from build123d import *

# Parameters (mm, degrees)
SKETCH_1_R          = 2.5
EXTRUDE_1_DEPTH     = 45
EXTRUDE_2_DEPTH     = 8
EXTRUDE_3_DEPTH     = 8
CHAMFER_1_SIZE      = 1
SKETCH_4_R          = 1.25
CUT_EXTRUDE_1_DEPTH = 8
CUT_EXTRUDE_START   = 8
SKETCH_5_R          = 1.25
CUT_EXTRUDE_2_DEPTH = 8


with BuildPart() as part:
    # 草图1 → 凸台-拉伸1 (new body)
    with BuildSketch(Plane(origin=(0, 0, 0), x_dir=(1, 0, 0), z_dir=(0, 1, 0))):
        with Locations(Location((0, 0, 0), (0, 0, 90))):
            Circle(SKETCH_1_R)
    extrude(amount=EXTRUDE_1_DEPTH)

    # 草图2 → 凸台-拉伸2 (add)
    with BuildSketch(Plane(origin=(0, 45, 0), x_dir=(1, 0, 0), z_dir=(0, 1, 0))):
        Polygon((3.202903935, -1.319623577), (2.744279509, 2.113984385), (-0.458624426, 3.433607962), (-3.202903935, 1.319623577), (-2.744279509, -2.113984385), (0.458624426, -3.433607962), align=None)
    extrude(amount=-EXTRUDE_2_DEPTH)

    # 草图3 → 凸台-拉伸3 (add)
    with BuildSketch(Plane.XZ):
        Polygon((3.202903935, 1.319623577), (0.458624426, 3.433607962), (-2.744279509, 2.113984385), (-3.202903935, -1.319623577), (-0.458624426, -3.433607962), (2.744279509, -2.113984385), align=None)
    extrude(amount=-EXTRUDE_3_DEPTH)

    # 倒角1
    # the kernel refuses this chamfer: 1 mm, written as the material it adds along each edge
    with BuildSketch(Plane(origin=(0, 37, 0), x_dir=(0, 0, -1), z_dir=(-1, 0, 0))) as chamfer_1_piece_1_section:
        Polygon((2.5, CHAMFER_1_SIZE), (2.5 + CHAMFER_1_SIZE, 0), (2.5, 0), align=None)
    chamfer_1_piece_1 = revolve(axis=Axis((0, 37, 0), (0, -1, 0)), mode=Mode.PRIVATE)
    chamfer_1_piece_1 = split(chamfer_1_piece_1, bisect_by=Plane(origin=(3.361202761, 36.482096178, 2.504767848), z_dir=(-0.9911972405355005, 0, 0.13239346794615373)), keep=Keep.TOP, mode=Mode.PRIVATE)
    chamfer_1_piece_1 = split(chamfer_1_piece_1, bisect_by=Plane(origin=(0.402796537, 36.482096178, 3.476613525), z_dir=(-0.61025472680424, 0, -0.7922052564917015)), keep=Keep.TOP, mode=Mode.PRIVATE)
    chamfer_1_piece_1 = split(chamfer_1_piece_1, bisect_by=Plane(origin=(2.183184145, 36.482096178, -2.345160432), z_dir=(-0.3809425137312606, 0, 0.924598724437855)), keep=Keep.TOP, mode=Mode.PRIVATE)
    chamfer_1_piece_1 = split(chamfer_1_piece_1, bisect_by=Plane(origin=(-0.102470937, 36.482096178, 3.202431915), z_dir=(0.38094251373126053, 0, -0.924598724437855)), keep=Keep.TOP, mode=Mode.PRIVATE)
    chamfer_1_piece_1 = split(chamfer_1_piece_1, bisect_by=Plane(origin=(-3.258731824, 36.482096178, -1.276618014), z_dir=(0.6102547268042401, 0, 0.7922052564917015)), keep=Keep.TOP, mode=Mode.PRIVATE)
    chamfer_1_piece_1 = split(chamfer_1_piece_1, bisect_by=Plane(origin=(-2.585980682, 36.482096178, 3.299128656), z_dir=(0.9911972405355005, 0, -0.1323934679461537)), keep=Keep.TOP, mode=Mode.PRIVATE)
    add(chamfer_1_piece_1)
    with BuildSketch(Plane(origin=(0, 8, 0), x_dir=(0, 0, -1), z_dir=(-1, 0, 0))) as chamfer_1_piece_2_section:
        Polygon((2.5 + CHAMFER_1_SIZE, 0), (2.5, -CHAMFER_1_SIZE), (2.5, 0), align=None)
    chamfer_1_piece_2 = revolve(axis=Axis((0, 8, 0), (0, -1, 0)), mode=Mode.PRIVATE)
    chamfer_1_piece_2 = split(chamfer_1_piece_2, bisect_by=Plane(origin=(0.402796537, 8.517903822, 3.476613525), z_dir=(-0.61025472680424, 0, -0.7922052564917015)), keep=Keep.TOP, mode=Mode.PRIVATE)
    chamfer_1_piece_2 = split(chamfer_1_piece_2, bisect_by=Plane(origin=(3.361202761, 8.517903822, 2.504767848), z_dir=(-0.9911972405355005, 0, 0.13239346794615373)), keep=Keep.TOP, mode=Mode.PRIVATE)
    chamfer_1_piece_2 = split(chamfer_1_piece_2, bisect_by=Plane(origin=(-0.102470937, 8.517903822, 3.202431915), z_dir=(0.38094251373126053, 0, -0.924598724437855)), keep=Keep.TOP, mode=Mode.PRIVATE)
    chamfer_1_piece_2 = split(chamfer_1_piece_2, bisect_by=Plane(origin=(2.183184145, 8.517903822, -2.345160432), z_dir=(-0.3809425137312606, 0, 0.924598724437855)), keep=Keep.TOP, mode=Mode.PRIVATE)
    chamfer_1_piece_2 = split(chamfer_1_piece_2, bisect_by=Plane(origin=(-2.585980682, 8.517903822, 3.299128656), z_dir=(0.9911972405355005, 0, -0.1323934679461537)), keep=Keep.TOP, mode=Mode.PRIVATE)
    chamfer_1_piece_2 = split(chamfer_1_piece_2, bisect_by=Plane(origin=(-3.258731824, 8.517903822, -1.276618014), z_dir=(0.6102547268042401, 0, 0.7922052564917015)), keep=Keep.TOP, mode=Mode.PRIVATE)
    add(chamfer_1_piece_2)

    # 草图4 → 切除-拉伸1 (cut)
    with BuildSketch(Plane(origin=(0, 0, 0), x_dir=(-1, 0, 0), z_dir=(0, 1, 0))):
        with Locations(Location((0, 0, 0), (0, 0, 90))):
            Circle(SKETCH_4_R)
    extrude(amount=CUT_EXTRUDE_1_DEPTH, mode=Mode.SUBTRACT)

    # 草图5 → 切除-拉伸2 (cut)
    with BuildSketch(Plane(origin=(0, 45, 0), x_dir=(-1, 0, 0), z_dir=(0, -1, 0)).offset(CUT_EXTRUDE_START)):
        with Locations(Location((0, 0, 0), (0, 0, 270))):
            Circle(SKETCH_5_R)
    extrude(amount=-CUT_EXTRUDE_2_DEPTH, mode=Mode.SUBTRACT)


solid = part.part
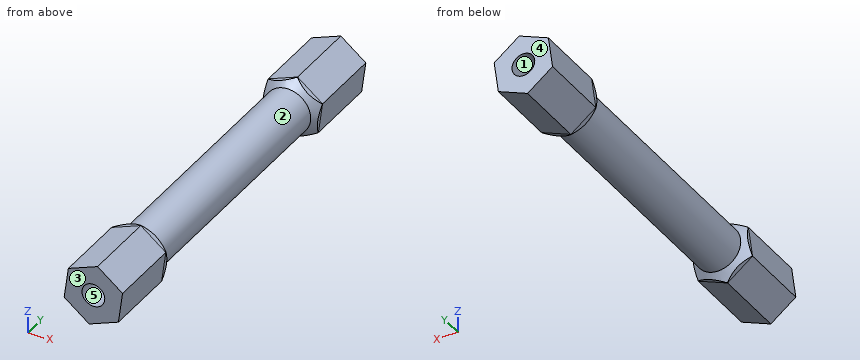
Design review of the part built by this model. Coordinates are the model's own, in mm. Face numbers are marked on the shaded views. A direction names the side the tool comes from. Give positions to 0.01 mm unless a question says otherwise; leave off trailing zeros. Write each loop counter-clockwise with the first axis right and the second up, starting at its lowest first coordinate (ties: lowest second). Pieces come first, ordered by that corner, then holes. Notation, with made-up numbers: M 74,42.5 L 131,42.5 A25 ccw 131,68.5 Z; hole C -7.75,14.5 d9. An arc over 180 degrees is marked long. Return JSON: item names as keys, results as strings. Group by question number.
Item 1: Take a section at B-B (x = 0). Give the boundary of the cut face in (y, z).
Item 2: Take a section at C-C (z = 0). Give the boundary of the cut face in (x, y), plus the area to 3 significant figures.
Item 3: The part is to be moulded in two halves that separate along X. For the marked faces 1, 2 and 3, say which applies: pulls with the +X half, pulls with the -X half, needs draft (parallel to the pull), parting line crosses it, or undercut.
Item 4: Clearance check with flat-ended pins moving along their axes: pin 1 Ø1.5 at (y, z) = (6, 1) entering from -X; pin 2 Ø2 at (x, z) = (0, 0) entering from +Y; pin 3 Ø3 at (x, y) = (0, 21.5) entering from +Z; pin 4 Ø3 at (x, z) = (0, 0) entering from -Y. State where each tip first meets the part, or that it passes through.
Item 5: Tool access review of the marked faces 4 and 5: name each direction out of +Z, -Z, +X, -X, +Y, -Y from which nothing blocks a thin tool from reaching the whole face with its end or side.
Item 6: Take a section at D-D (y = 19.5). Give the boundary of the cut face in (x, z), plus the area to 3 significant figures.
Item 7: Take a section at A-A (y = 7). Give the boundary of the cut face in (x, z), plus the area to 3 significant figures.
Item 8: Wall thickness on line 1 along X through (y, z) = (39.75, 0); line 2 along Y through (x, z) = (1, 0.5); line 3 along Y through (x, z) = (-2.5, 1.5): over which ranges is each line inside the solid? List them lowest first.
Return value:
{
 "1": {"outline": "M 0,-3.24 L 8.26,-3.24 L 9,-2.5 L 36,-2.5 L 36.74,-3.24 L 45,-3.24 L 45,-1.25 L 37,-1.25 L 37,1.25 L 45,1.25 L 45,3.24 L 36.74,3.24 L 36,2.5 L 9,2.5 L 8.26,3.24 L 0,3.24 L 0,1.25 L 8,1.25 L 8,-1.25 L 0,-1.25 Z"},
 "2": {"outline": "M -3.03,0 L -1.25,0 L -1.25,8 L 1.25,8 L 1.25,0 L 3.03,0 L 3.03,8.47 L 2.5,9 L 2.5,36 L 3.03,36.53 L 3.03,45 L 1.25,45 L 1.25,37 L -1.25,37 L -1.25,45 L -3.03,45 L -3.03,36.53 L -2.5,36 L -2.5,9 L -3.03,8.47 Z", "area": "203 mm2"},
 "3": {"face 1": "undercut", "face 2": "parting line crosses it", "face 3": "needs draft"},
 "4": {"pin 1": "stops at x = -2.99", "pin 2": "stops at y = 37", "pin 3": "stops at z = 2.5", "pin 4": "stops at y = 0"},
 "5": {"face 4": "+Z, -Z, +X, -X, +Y", "face 5": "-Y"},
 "6": {"outline": "C 0,0 d5", "area": "19.6 mm2"},
 "7": {"outline": "M -3.2,-1.32 L -0.46,-3.43 L 2.74,-2.11 L 3.2,1.32 L 0.46,3.43 L -2.74,2.11 Z; hole C 0,0 d2.5", "area": "26.3 mm2"},
 "8": {"line 1": "x = -3.03 to -1.25, 1.25 to 3.03", "line 2": "y = 8 to 37", "line 3": "y = 0 to 8.58, 36.42 to 45"}
}
